The figure shows three views and two pictorial views of one solid part (mm, origin at its lowest corner). Answer the questions. A direction names the side the tool comes from. Give positions to 0.01 mm unless a question says otherwise; leave off trailing zeros. Write each loop counter-clockwise with the first axis right and the second up, starting at its lowest first coordinate (ties: lowest second). Pieces come first, ordered by that corner, then holes. Notation, with made-up numbers: (73.25, 31) - (121.25, 31) arc R23 ccw to (121.25, 53) - close; hole circle Ø7 at (-16, 30). An arc over 180 degrees is marked (long way). One line per question, with ' | ' between items. Start each with the question number.
1. A cutting plane is placed at A-A (x = 11). Determine the outline of the cut face in (y, z), then the cut area to 3 significant figures.
2. A cutting plane is placed at B-B (z = 8.5). Determine the outline of the cut face in (x, y).
3. A cutting plane is placed at D-D (z = 1.5). Determine the outline of the cut face in (x, y).
4. The mould has two halves that part along Z. Classify the marked faces 1, 2 and 3: +Z half, -Z half, draft (parallel to the pull), parting line (faces both ways), or undercut.
5. For the marked faces 4 and 5, determine the directions among +Z, -Z, +X, -X, +Y, -Y from which every point of the face is accessible in a straight line to the end or side of a thin tool.
6. Find the intervals of material crossed by L1, parallel to Z at x = 8.25, y = 10.25; L2, parallel to X at y = 7.75, z = 6, in increasing order. Write a range as from..to.
7. Given P1, Ø7.5, axis at x = 8.5, y = 6.5, coming from the -Z side; P2, Ø3, axis at x = 13, y = 3, coming from the -Z side; P3, Ø3.5, axis at y = 10.21, z = 9.45, coming from the +X side, each flat-ended and moving along its own axis, determine where each tip first touches the part or whether it passes through.
8. A cutting plane is placed at C-C (y = 7.75). Determine the outline of the cut face in (x, z), then the cut area to 3 significant figures.
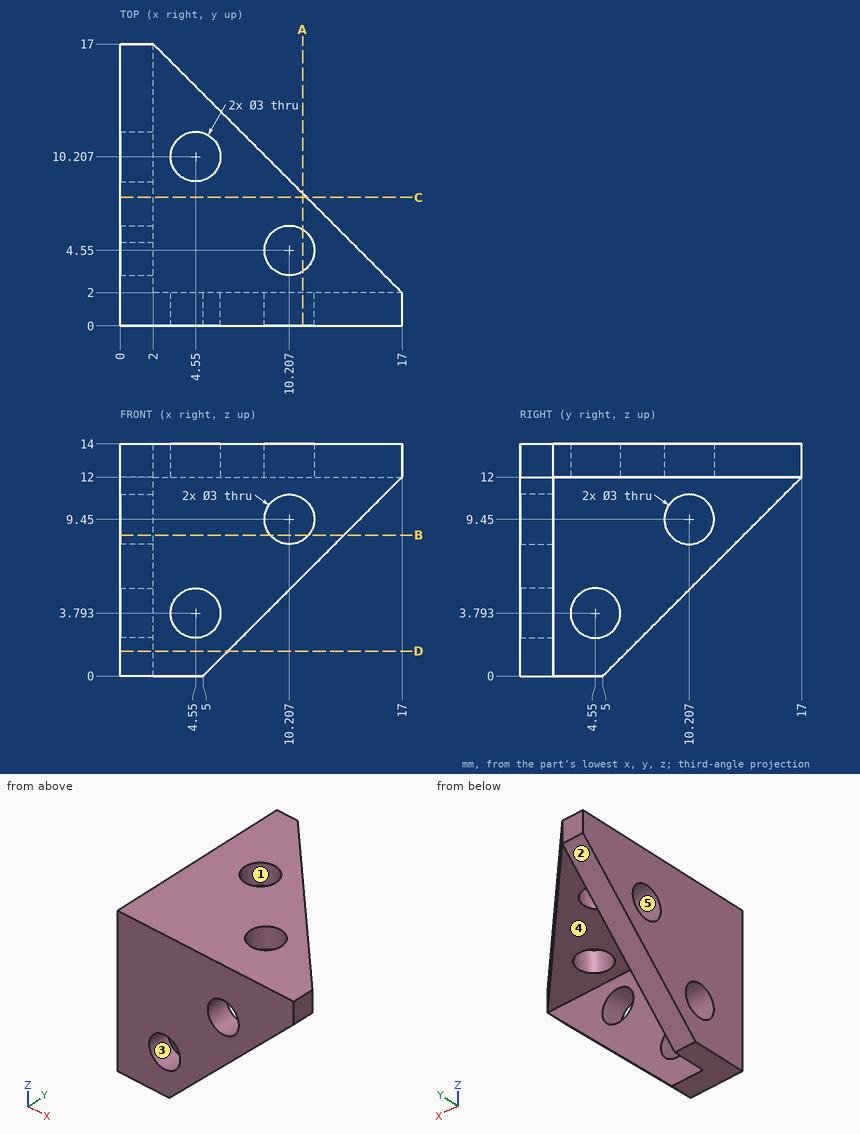
Determined:
1) outline: (0, 6) - (2, 6) - (2, 8.18) - (0, 8.18) - close; (0, 10.72) - (2, 10.72) - (2, 12) - (3.28, 12) - (3.28, 14) - (0, 14) - close; (5.82, 12) - (8, 12) - (8, 14) - (5.82, 14) - close | area: 17.8 mm2
2) outline: (0, 0) - (9.05, 0) - (9.05, 2) - (2, 2) - (2, 9.05) - (0, 9.05) - close; (0, 11.37) - (2, 11.37) - (2, 13.5) - (0, 13.5) - close; (11.37, 0) - (13.5, 0) - (13.5, 2) - (11.37, 2) - close
3) outline: (0, 0) - (6.5, 0) - (6.5, 2) - (2, 2) - (2, 6.5) - (0, 6.5) - close
4) face 1: draft | face 2: -Z half | face 3: undercut
5) face 4: -Z, +X, +Y | face 5: +X, -X
6) L1: 12..14 | L2: 0..2
7) P1: z = 12 | P2: z = 6.88 | P3: x = 2
8) outline: (0, 2.75) - (2, 2.75) - (2, 12) - (11.25, 12) - (11.25, 14) - (0, 14) - close | area: 41.0 mm2
